Source: three-view drawing plus pictorial views. Frame: mm from the lowest corner of the part. A direction names the side the tool comes from. Give positions to 0.01 mm unless a question says otherwise; leave off trailing zeros. Loops run counter-clockwise (first coordinate to the right, second up) from the corner with the lowest first, then second, coordinate; pieces in that order, holes last. Notation, with made-up numbers: (89.25, 80) - (113.25, 80) arc R12 cw to (113.25, 91) - close; hole circle Ø7 at (31, 76.5). An arc over 180 degrees is marked (long way). Answer as a JSON object with one key per item and string values.
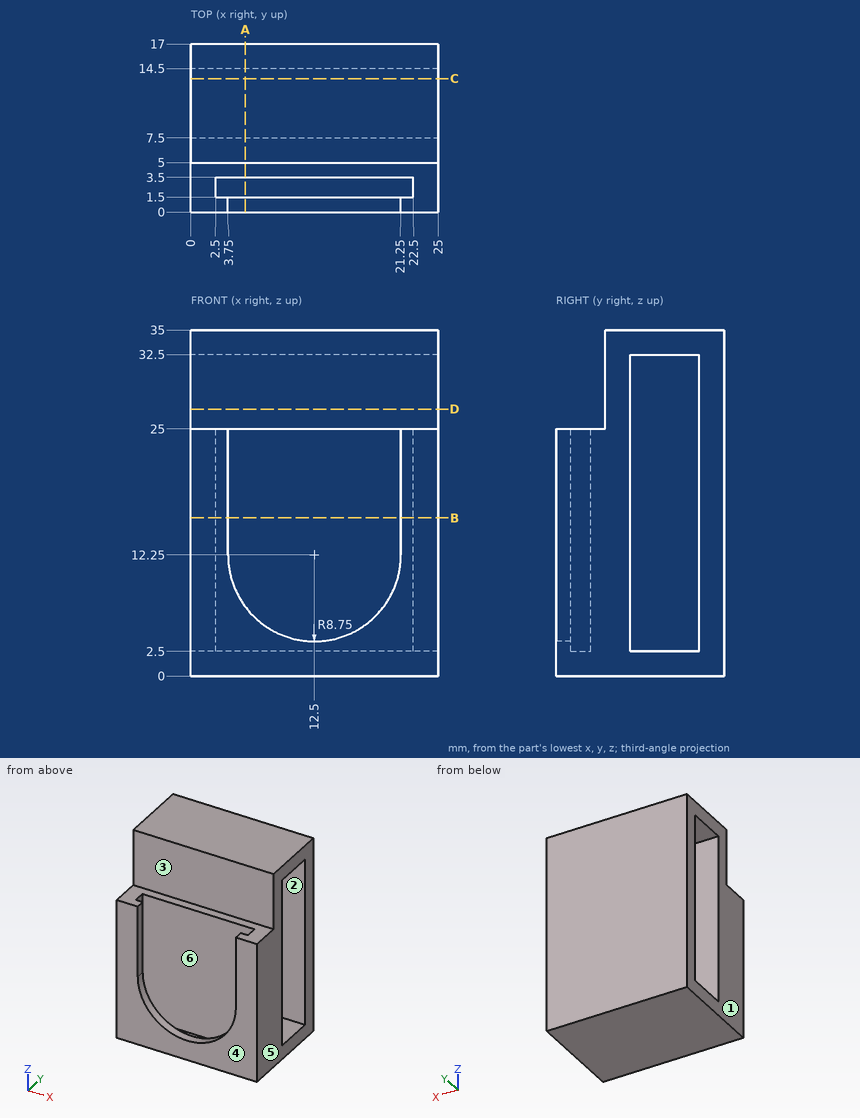
Item 1: Contact query for flat-ended pins moving along their axis: P1, Ø5, axis at x = 16.5, z = 24.5, coming from the -Y side; P2, Ø1, axis at x = 19.5, y = 5, coming from the -Z side; P3, Ø1.6, axis at x = 15, y = 2.5, coming from the +Z side; P4, Ø5.5, axis at x = 7, y = 1.5, coming from the +Z side. Output: stop coordinate, or through.
Geometry check:
{"P1": "stops at y = 3.5", "P2": "stops at z = 0", "P3": "stops at z = 2.5", "P4": "stops at z = 25"}
Item 2: Material intervals for line 1 (Y direction, x = 3, z = 20.5); line 2 (Y direction, x = 14, z = 22.5); line 3 (Z direction, x = 22, y = 10), sorted ascending. Write a range as [from, to].
Geometry check:
{"line 1": "y = [0, 1.5], [3.5, 7.5], [14.5, 17]", "line 2": "y = [3.5, 7.5], [14.5, 17]", "line 3": "z = [0, 2.5], [32.5, 35]"}
Item 3: Cut plane A-A (x = 5.5). Return loops of the section in (y, z).
Geometry check:
{"outline": "(0, 0) - (17, 0) - (17, 35) - (5, 35) - (5, 25) - (3.5, 25) - (3.5, 2.5) - (1.5, 2.5) - (1.5, 7) - (0, 7) - close; hole (7.5, 2.5) - (14.5, 2.5) - (14.5, 32.5) - (7.5, 32.5) - close"}
Item 4: Access query for the marked faces 1, 2 and 3. Directions: +Z, -Z, +X, -X, +Y, -Y. A direction counts if a zero-diameter tool reaches every point of the face in a straight line with its end or side. Return the directions, or none.
Geometry check:
{"face 1": "+Z, -Z, -X, +Y, -Y", "face 2": "+X, -X", "face 3": "+Z, +X, -X, -Y"}
Item 5: Mould query, pull axis X, two halves, no side actions, for the marked faces 4, 5 and 6. Classes: released by +X, released by -X, zero draft, split by the parting line, or undercut.
Geometry check:
{"face 4": "zero draft", "face 5": "released by +X", "face 6": "undercut"}
Item 6: Cut plane D-D (z = 27). Return loops of the section in (x, y), then the cut area to 3 significant figures.
Geometry check:
{"outline": "(0, 5) - (25, 5) - (25, 7.5) - (0, 7.5) - close; (0, 14.5) - (25, 14.5) - (25, 17) - (0, 17) - close", "area": "125 mm2"}
Item 7: Cut plane C-C (y = 13.5). Return loops of the section in (x, z).
Geometry check:
{"outline": "(0, 0) - (25, 0) - (25, 2.5) - (0, 2.5) - close; (0, 32.5) - (25, 32.5) - (25, 35) - (0, 35) - close"}
Item 8: Cut plane B-B (z = 16). Return loops of the section in (x, y), then the cut area to 3 significant figures.
Geometry check:
{"outline": "(0, 0) - (3.75, 0) - (3.75, 1.5) - (2.5, 1.5) - (2.5, 3.5) - (22.5, 3.5) - (22.5, 1.5) - (21.25, 1.5) - (21.25, 0) - (25, 0) - (25, 7.5) - (0, 7.5) - close; (0, 14.5) - (25, 14.5) - (25, 17) - (0, 17) - close", "area": "184 mm2"}
